```python
from build123d import *

# Parameters (mm, degrees)
SKETCH1_R           = 11.5
BOSS_EXTRUDE1_DEPTH = 19
SKETCH2_W           = 10
SKETCH2_H           = 4
BOSS_EXTRUDE2_DEPTH = 4
SKETCH3_R           = 3.5
SKETCH3_R_2         = 1.25
CUT_EXTRUDE1_DEPTH  = 9


with BuildPart() as part:
    # Sketch1 → Boss-Extrude1 (new body)
    with BuildSketch(Plane(origin=(0, 0, 0), x_dir=(1, 0, 0), z_dir=(0, 1, 0))):
        with Locations(Location((0, 0, 0), (0, 0, 270))):
            Circle(SKETCH1_R)
    extrude(amount=BOSS_EXTRUDE1_DEPTH)

    # Sketch2 → Boss-Extrude2 (add)
    with BuildSketch(Plane(origin=(0, 19, 0), x_dir=(1, 0, 0), z_dir=(0, 1, 0))):
        with Locations((0, -5)):
            Rectangle(SKETCH2_W, SKETCH2_H)
    extrude(amount=BOSS_EXTRUDE2_DEPTH)

    # Sketch3 → Cut-Extrude1 (cut)
    with BuildSketch(Plane.XZ):
        with Locations(Location((0, 0, 0), (0, 0, 270))):
            Circle(SKETCH3_R)
        with Locations(Location((0, 8.5, 0), (0, 0, 270))):
            Circle(SKETCH3_R_2)
        with Locations(Location((0, -8.5, 0), (0, 0, 270))):
            Circle(SKETCH3_R_2)
    extrude(amount=-CUT_EXTRUDE1_DEPTH, mode=Mode.SUBTRACT)


solid = part.part
```
Work out the finished part from the listing and answer in its coordinate system (mm). A direction names the side the tool comes from. Coordinates: 2 decimals unless noted, no trailing zeros. Write each loop counter-clockwise with the first axis right and the second up, starting at its lowest first coordinate (ties: lowest second). Pieces come first, ordered by that corner, then holes.
Q1. A cutting plane is placed at A-A, the plane x = 0. Give the vertices of the cut face in (y, z).
Q2. A cutting plane is placed at B-B, the plane z = 0. Give the vertices of the cut face in (x, y), then the cut area to 3 significant figures.
Q3. A cutting plane is placed at C-C, the plane y = 15.25. Give the vertices of the cut face in (x, z).
Q4. Each of these flat-tipped pins is pushed along its axis until it touches: pin 1 Ø2 at (x, y) = (-2, 21) entering from +Z; pin 2 Ø3 at (x, y) = (2, 21) entering from -Z; pin 3 Ø6 at (x, y) = (-3.5, 18.5) entering from +Z. Where does it stop, or does it pass through?
Q5. Determine the mould class of faces 1 (the face through (0, 9, 9)), 2 (the face through (-5, 21, 5)), 3 (the face through (0.05, 4.44, -7.25)), 4 (the face through (0, 21, 3)) for opening direction X: released by +X, released by -X, zero draft, split by the parting line, or undercut.
Q6. Which of the six approach directions +Z, -Z, +X, -X, +Y, -Y give full straight-line access (tool end or side, diameter ignored) to faces 5 (the face through (5, 21, 5)), 6 (the face through (0, 21, 7)), 7 (the face through (0.05, 4.44, 9.75))?
Q7. Find the intervals of material crossed by line 1 (Y direction, x = -1.5, z = -4); line 2 (Z direction, x = -4.75, y = 22); line 3 (X direction, y = 6.5, z = 8.5), in increasing order.
Q8. A cutting plane is placed at D-D, the plane z = -8.5. Give the vertices of the cut face in (x, y).
Findings below:
1. outline: (0, -11.5) - (19, -11.5) - (19, 3) - (23, 3) - (23, 7) - (19, 7) - (19, 11.5) - (0, 11.5) - (0, 9.75) - (9, 9.75) - (9, 7.25) - (0, 7.25) - (0, 3.5) - (9, 3.5) - (9, -3.5) - (0, -3.5) - (0, -7.25) - (9, -7.25) - (9, -9.75) - (0, -9.75) - close
2. outline: (-11.5, 0) - (-3.5, 0) - (-3.5, 9) - (3.5, 9) - (3.5, 0) - (11.5, 0) - (11.5, 19) - (-11.5, 19) - close
2. area: 374 mm2
3. outline: circle Ø23 at (0, 0)
4. pin 1: stops at z = 7
4. pin 2: stops at z = 3
4. pin 3: stops at z = 11.49
5. face 1: undercut
5. face 2: released by -X
5. face 3: undercut
5. face 4: zero draft
6. face 5: +Z, -Z, +X, +Y
6. face 6: +Z, +X, -X, +Y
6. face 7: -Y
7. line 1: y = 0 to 19
7. line 2: z = 3 to 7
7. line 3: x = -7.75 to -1.25, 1.25 to 7.75
8. outline: (-7.75, 0) - (-1.25, 0) - (-1.25, 9) - (1.25, 9) - (1.25, 0) - (7.75, 0) - (7.75, 19) - (-7.75, 19) - close
